from build123d import *

# Parameters (mm, degrees)
CROQUIS1_R              = 9.875
CROQUIS1_W              = 5
CROQUIS1_H              = 5
SALIENTE_EXTRUIR1_DEPTH = 3
REDONDEO1_R             = 1
CROQUIS2_R              = 10.5
CORTAR_EXTRUIR1_DEPTH   = 10
CROQUIS3_W              = 19.75
CROQUIS3_H              = 2
SALIENTE_EXTRUIR2_DEPTH = 11
REDONDEO2_R             = 1


with BuildPart() as part:
    # Croquis1 → Saliente-Extruir1 (new body)
    with BuildSketch(Plane.XY):
        Circle(CROQUIS1_R)
        with BuildLine():
            ThreePointArc((9.875, 0), (0, -9.875), (-9.875, 0))
            Line((-9.875, 0), (-9.875, -10.4))
            Line((-9.875, -10.4), (-9.875, -15.4))
            Line((-9.875, -15.4), (-9.875, -25.4))
            Line((-9.875, -25.4), (9.875, -25.4))
            Line((9.875, -25.4), (9.875, -15.4))
            Line((9.875, -15.4), (9.875, -10.4))
            Line((9.875, -10.4), (9.875, 0))
        make_face()
        with Locations((12.375, -12.9)):
            Rectangle(CROQUIS1_W, CROQUIS1_H)
        with Locations((-12.375, -12.9)):
            Rectangle(CROQUIS1_W, CROQUIS1_H)
    extrude(amount=SALIENTE_EXTRUIR1_DEPTH)

    # Redondeo1
    redondeo1_edges = [part.edges().sort_by_distance(p)[0] for p in [
        (0, -25.4, 3),
    ]]
    fillet(redondeo1_edges, radius=REDONDEO1_R)

    # Croquis2 → Cortar-Extruir1 (cut)
    with BuildSketch(Plane.XY.offset(3)):
        Circle(CROQUIS2_R)
    extrude(amount=-CORTAR_EXTRUIR1_DEPTH, mode=Mode.SUBTRACT)

    # Croquis3 → Saliente-Extruir2 (add)
    with BuildSketch(Plane(origin=(0, 0, 0), x_dir=(-1, 0, 0), z_dir=(0, 0, -1))):
        with Locations((0, -24.4)):
            Rectangle(CROQUIS3_W, CROQUIS3_H)
    extrude(amount=SALIENTE_EXTRUIR2_DEPTH)

    # Redondeo2
    redondeo2_edges = [part.edges().sort_by_distance(p)[0] for p in [
        (0, -23.4, 0),
    ]]
    fillet(redondeo2_edges, radius=REDONDEO2_R)


solid = part.part
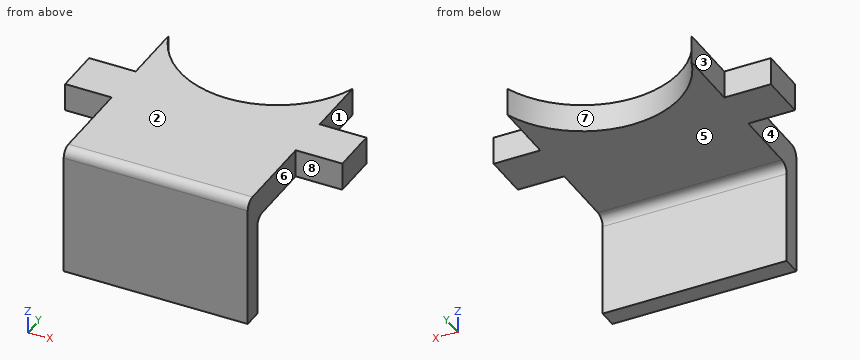
Work out the finished part from the listing and answer in its coordinate system (mm). Face numbers are marked on the shaded views. A direction names the side the tool comes from. Coordinates: 2 decimals unless noted, no trailing zeros. Write each loop counter-clockwise with the first axis right and the second up, starting at its lowest first coordinate (ties: lowest second). Pieces come first, ordered by that corner, then holes.
1. The part is cut by section C-C, the plane z = -7.5. Write down the section's boundary in (x, y) (3 decimals), and give its area (3 significant figures).
Results list:
outline: (-9.875, -25.4) - (9.875, -25.4) - (9.875, -23.4) - (-9.875, -23.4) - close
area: 39.5 mm2
2. For the marked faces 1, 2, 3, 4 and 5, determine the directions among +Z, -Z, +X, -X, +Y, -Y from which every point of the face is accessible in a straight line to the end or side of a thin tool.
Results list:
face 1: +Z, -Z, +X, +Y
face 2: +Z, +X, -X, +Y, -Y
face 3: +Z, -Z, -X, +Y
face 4: +Z, -Z, -X, -Y
face 5: -Z, +X, -X, +Y
3. For a pull along X with two mould halves and no side action, classify the marked faces 6, 7 and 8 as +X half, -X half, draft (parallel to the pull), parting line (faces both ways), or undercut.
Results list:
face 6: +X half
face 7: undercut
face 8: draft
4. Consider line 1 along Y through (x, z) = (2.5, -1.75); line 2 along Z through (x, y) = (8.5, -11.5); line 3 along X through (y, z) = (-23.5, -10.25) (3 decimals). Determine where each line is inside the solid, lowest interval first.
Results list:
line 1: y = -25.4 to -23.4
line 2: z = 0 to 3
line 3: x = -9.875 to 9.875
5. Flat-ended cylindrical pins translate along their axes: pin 1 (1.5 mm diameter, centred on y = -7.5, z = 1, fed in from +X) (3 decimals); pin 2 (3 mm diameter, centred on x = -5, z = -4, fed in from +Y); pin 3 (1.5 mm diameter, centred on x = 12, z = 1.5, fed in from -Y). Find the tip coordinate at first contact, or state that the pin passes through.
Results list:
pin 1: stops at x = 9.875
pin 2: stops at y = -23.4
pin 3: stops at y = -15.4
6. The part is cut by section D-D, the plane y = -7.75. Write down the section's boundary in (x, z) (3 decimals), and give its area (3 significant figures).
Results list:
outline: (-9.875, 0) - (-7.084, 0) - (-7.084, 3) - (-9.875, 3) - close; (7.084, 0) - (9.875, 0) - (9.875, 3) - (7.084, 3) - close
area: 16.7 mm2
7. The part is cut by section A-A, the plane y = -5.5. Write down the section's boundary in (x, z) (3 decimals).
Results list:
outline: (-9.875, 0) - (-8.944, 0) - (-8.944, 3) - (-9.875, 3) - close; (8.944, 0) - (9.875, 0) - (9.875, 3) - (8.944, 3) - close
8. The part is cut by section B-B, the plane x = 3.25. Write down the section's boundary in (y, z), and give its area (3 significant figures).
Results list:
outline: (-25.4, -11) - (-23.4, -11) - (-23.4, -1) arc R1 cw to (-22.4, 0) - (-9.98, 0) - (-9.98, 3) - (-24.4, 3) arc R1 ccw to (-25.4, 2) - close
area: 68.2 mm2
